Geometry check sheet. Reference: drawing and pictorial views, mm from the part's lowest x, y, z. A direction names the side the tool comes from. Give positions to 0.01 mm unless a question says otherwise; leave off trailing zeros. Write each loop counter-clockwise with the first axis right and the second up, starting at its lowest first coordinate (ties: lowest second). Pieces come first, ordered by that corner, then holes. Notation, with made-up numbers: M 25.5,84 L 58.5,84 A17 cw 58.5,105 Z; hole C -24,47.5 d10. An arc over 180 degrees is marked long. Answer as a JSON object with one key per item and string values.
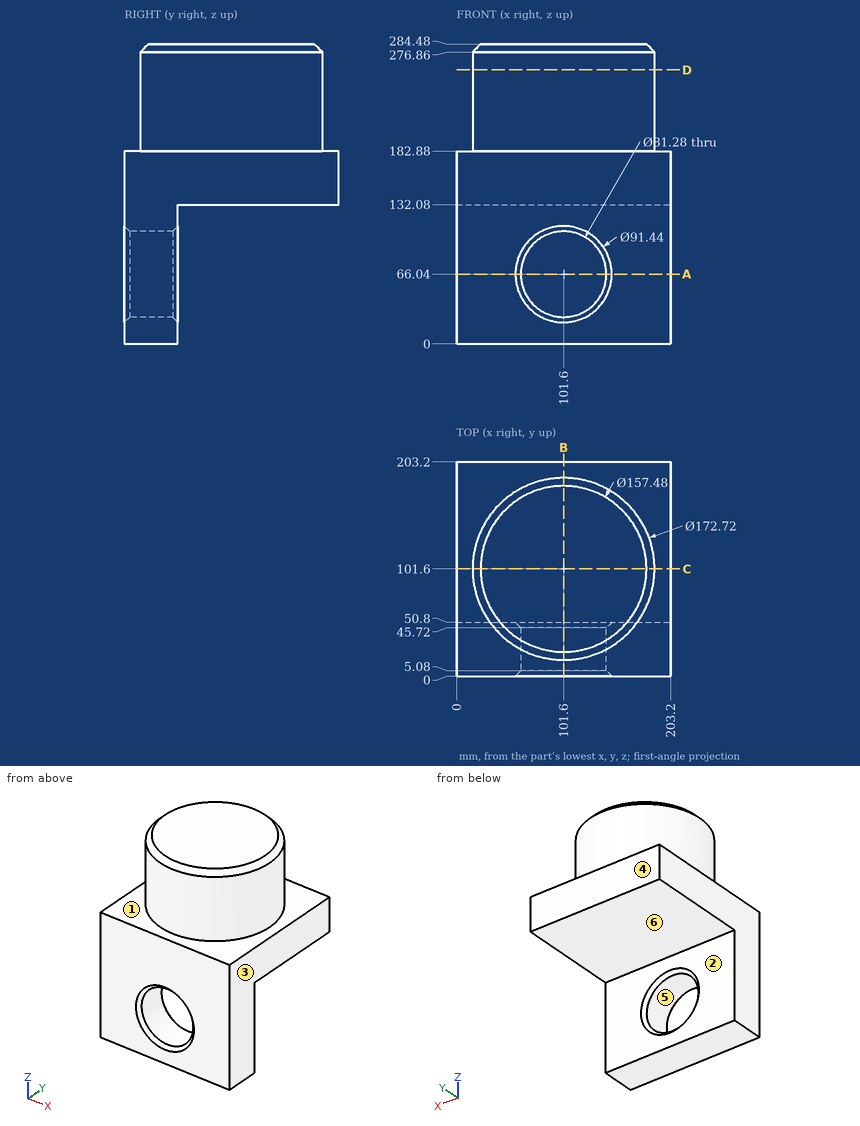
1) Access from +Z, -Z, +X, -X, +Y, -Y to the whole of each face (thin tool, end or side, straight path). Record for the marked faces 1, 2 and 3.
Completed:
{"face 1": "+Z", "face 2": "-Z, +X, -X, +Y", "face 3": "+Z, -Z, +X, +Y, -Y"}
2) Section check A-A on z = 66.04. Record the boundary of the cut face in (x, y), and give its area (3 significant figures).
Completed:
{"outline": "M 0,0 L 55.88,0 L 60.96,5.08 L 60.96,45.72 L 55.88,50.8 L 0,50.8 Z; M 142.24,5.08 L 147.32,0 L 203.2,0 L 203.2,50.8 L 147.32,50.8 L 142.24,45.72 Z", "area": "6,140 mm2"}
3) Section check C-C on y = 101.6. Record the boundary of the cut face in (x, z), and give its area (3 significant figures).
Completed:
{"outline": "M 0,132.08 L 203.2,132.08 L 203.2,182.88 L 187.96,182.88 L 187.96,276.86 L 180.34,284.48 L 22.86,284.48 L 15.24,276.86 L 15.24,182.88 L 0,182.88 Z", "area": "27,800 mm2"}
4) Release check for a two-part mould opening along Z. For the marked faces 4, 5 and 6 record: pulls with the +Z half, pulls with the -Z half, needs draft (parallel to the pull), parting line crosses it, or undercut.
Completed:
{"face 4": "needs draft", "face 5": "undercut", "face 6": "pulls with the -Z half"}
5) Go/stop test with flat-tipped pins: pin 1 (3 mm diameter, centred on x = 51, z = 215, fed in from -Y); pin 2 (12 mm diameter, centred on y = 60.5, z = 124.5, fed in from +X); pin 3 (5 mm diameter, centred on y = 130.5, z = 245.5, fed in from +X); pin 4 (6 mm diameter, centred on x = 73.5, z = 125.5, fed in from +Y). Record where each tip stops, or that it passes through.
Completed:
{"pin 1": "stops at y = 30.56", "pin 2": "passes through", "pin 3": "stops at x = 183.83", "pin 4": "stops at y = 50.8"}
6) Section check D-D on z = 260. Record the boundary of the cut face in (x, y).
Completed:
{"outline": "C 101.6,101.6 d172.72"}
7) Section check B-B on x = 101.6. Record the boundary of the cut face in (y, z).
Completed:
{"outline": "M 0,0 L 50.8,0 L 50.8,20.32 L 45.72,25.4 L 5.08,25.4 L 0,20.32 Z; M 0,111.76 L 5.08,106.68 L 45.72,106.68 L 50.8,111.76 L 50.8,132.08 L 203.2,132.08 L 203.2,182.88 L 187.96,182.88 L 187.96,276.86 L 180.34,284.48 L 22.86,284.48 L 15.24,276.86 L 15.24,182.88 L 0,182.88 Z"}
8) Thickness scan on L1, parallel to Z at x = 101, y = 27; L2, parallel to X at y = 32, z = 66; L3, parallel to Z at x = 74.5, y = 192.5. Record the ranges inside material, lowest first.
Completed:
{"L1": "z = 0 to 25.4, 106.68 to 284.48", "L2": "x = 0 to 60.96, 142.24 to 203.2", "L3": "z = 132.08 to 182.88"}
